Check sheet for the modelled part. Datum: model origin and axes. Units: mm. A direction names the side the tool comes from. Round coordinates to 2 decimals unless told otherwise and drop trailing zeros. Write each loop counter-clockwise with the first axis right and the second up, starting at its lowest first coordinate (ties: lowest second). Pieces come first, ordered by that corner, then holes. Notation, with made-up numbers: M 30,12.5 L 85,12.5 A24 cw 85,35.5 Z; hole C -16.5,24.5 d11. An arc over 180 degrees is marked long. Put each result on its own line as item: value.
```python
from build123d import *

# Parameters (mm, degrees)
SKETCH1_R           = 40
SKETCH1_R_2         = 2.85
SKETCH1_R_3         = 5
SKETCH1_R_4         = 56.3
SKETCH1_R_5         = 2.95
BOSS_EXTRUDE1_DEPTH = 26
CUT_EXTRUDE1_DEPTH  = 24.2


with BuildPart() as part:
    # Sketch1 → Boss-Extrude1 (new body)
    with BuildSketch(Plane(origin=(0, 0, 0), x_dir=(1, 0, 0), z_dir=(0, 1, 0))):
        with BuildLine():
            Line((226.010043478, 56.158438787), (-2.834782609, 39.899423649))
            ThreePointArc((-2.834782609, 39.899423649), (27.263608489, 29.269363713), (40, 0))
            ThreePointArc((40, 0), (27.263608489, -29.269363713), (-2.834782609, -39.899423649))
            Line((-2.834782609, -39.899423649), (226.010043478, -56.158438787))
            ThreePointArc((226.010043478, -56.158438787), (173.7, 0), (226.010043478, 56.158438787))
        make_face()
        Circle(SKETCH1_R)
        with Locations((-27.35, 0)):
            Circle(SKETCH1_R_2, mode=Mode.SUBTRACT)
        with Locations((0, -27.35)):
            Circle(SKETCH1_R_2, mode=Mode.SUBTRACT)
        with Locations((27.35, 0)):
            Circle(SKETCH1_R_2, mode=Mode.SUBTRACT)
        with Locations((0, 27.35)):
            Circle(SKETCH1_R_2, mode=Mode.SUBTRACT)
        Circle(SKETCH1_R_3, mode=Mode.SUBTRACT)
        with Locations((230, 0)):
            Circle(SKETCH1_R_4)
        with Locations((195.05, 0)):
            Circle(SKETCH1_R_5, mode=Mode.SUBTRACT)
        with Locations((230, -34.95)):
            Circle(SKETCH1_R_5, mode=Mode.SUBTRACT)
        with Locations((264.95, 0)):
            Circle(SKETCH1_R_5, mode=Mode.SUBTRACT)
        with Locations((230, 34.95)):
            Circle(SKETCH1_R_5, mode=Mode.SUBTRACT)
        with Locations((230, 0)):
            Circle(SKETCH1_R_3, mode=Mode.SUBTRACT)
    extrude(amount=BOSS_EXTRUDE1_DEPTH)

    # Sketch2 → Cut-Extrude1 (cut)
    with BuildSketch(Plane(origin=(0, 26, 0), x_dir=(1, 0, 0), z_dir=(0, 1, 0))):
        with BuildLine():
            Line((-2.721391304, -38.303446704), (226.123434783, -54.562461841))
            ThreePointArc((226.123434783, -54.562461841), (284.7, 0), (226.123434783, 54.562461841))
            Line((226.123434783, 54.562461841), (-2.721391304, 38.303446704))
            ThreePointArc((-2.721391304, 38.303446704), (-38.4, 0), (-2.721391304, -38.303446704))
        make_face()
    extrude(amount=-CUT_EXTRUDE1_DEPTH, mode=Mode.SUBTRACT)


solid = part.part
```
1. Access from +Z, -Z, +X, -X, +Y, -Y to the whole of each face (thin tool, end or side, straight path). Record for faces 1 (the flat face through (113.19, 12.818, -48.143)), 2 (the flat face through (113.303, 14.069, -46.547)).
Computed values:
face 1: -Z, -X, +Y, -Y
face 2: +Y
2. Cross-section at A-A (y = 7.5). Enter the section's corners in (x, z), then the cut area to 3 significant figures.
Computed values:
outline: M -2.83,-39.9 L 226.01,-56.16 A56.3 ccw long 226.01,56.16 L -2.83,39.9 A40 ccw Z; hole M -2.72,-38.3 L 226.12,-54.56 A54.7 ccw long 226.12,54.56 L -2.72,38.3 A38.4 ccw Z
area: 1,210 mm2
3. Release check for a two-part mould opening along X. For faces 3 (the cylindrical face through (232.814, 0.887, -35.836)), 4 (the cylindrical face through (-39.99, 12.82, -0.84)), 5 (the flat face through (147, 26, 50)) record: +X half, -X half, draft (parallel to the pull), parting line (faces both ways), or undercut.
Computed values:
face 3: undercut
face 4: -X half
face 5: draft
4. Cross-section at B-B (x = 195.05). Enter the section's corners in (y, z), then the cut area to 3 significant figures.
Computed values:
outline: M 0,-53.96 L 26,-53.96 L 26,-52.35 L 1.8,-52.35 L 1.8,-2.95 L 0,-2.95 Z; M 0,2.95 L 1.8,2.95 L 1.8,52.35 L 26,52.35 L 26,53.96 L 0,53.96 Z
area: 261 mm2
5. Cross-section at C-C (z = 27.35). Enter the section's corners in (x, y), then the cut area to 3 significant figures.
Computed values:
outline: M -29.19,0 L -2.85,0 L -2.85,1.8 L -26.95,1.8 L -26.95,26 L -29.19,26 Z; M 2.85,0 L 279.21,0 L 279.21,26 L 277.37,26 L 277.37,1.8 L 2.85,1.8 Z
area: 643 mm2
6. Cross-section at D-D (x = 242.5). Enter the section's corners in (y, z), then the cut area to 3 significant figures.
Computed values:
outline: M 0,-54.89 L 26,-54.89 L 26,-53.25 L 1.8,-53.25 L 1.8,53.25 L 26,53.25 L 26,54.89 L 0,54.89 Z
area: 277 mm2
7. Scan lines: probe 1 along Z at (x, y) = (230, 0.55); probe 2 along X at (y, z) = (9.25, 2); probe 3 along X at (y, z) = (15.75, -1). Record each from-to range of solid material in increasing order.
Computed values:
probe 1: z = -56.3 to -37.9, -32 to -5, 5 to 32, 37.9 to 56.3
probe 2: x = -39.95 to -38.35, 284.66 to 286.26
probe 3: x = -39.99 to -38.39, 284.69 to 286.29
8. Depth check by flat-ended pin: pin 1 Ø9 at (x, z) = (230, 0) entering from +Y; pin 2 Ø3 at (y, z) = (23.5, 7) entering from +X; pin 3 Ø6 at (y, z) = (9.5, -15) entering from -X; pin 4 Ø2 at (x, y) = (137.5, 22.5) entering from +Z. Enter the tip coordinate at first touch or a pass-through.
Computed values:
pin 1: passes through
pin 2: stops at x = 286.03
pin 3: stops at x = -38.16
pin 4: stops at z = 49.94
